Geometry: final body of the model. Coordinates: model frame, mm. Face numbers are marked on the shaded views. A direction names the side the tool comes from. Give positions to 0.01 mm unless a question says otherwise; leave off trailing zeros. Write each loop counter-clockwise with the first axis right and the second up, starting at its lowest first coordinate (ties: lowest second). Pieces come first, ordered by that corner, then holes. Notation, with made-up numbers: M 61.5,9 L 97.5,9 A34 cw 97.5,47 Z; hole C -18,0.25 d9. An arc over 180 degrees is marked long. Use a Markdown table: item, result. Add a question column.
1) Section A-A on x = 5. Return the cut outline in (y, z), then the cut area to 3 significant figures.
2) Section B-B on z = 5.5. Return the cut outline in (x, y).
3) Section C-C on x = -5.5. Return the cut outline in (y, z), then the cut area to 3 significant figures.
4) Line query: line 1 (Z direction, x = 5, y = 2.25); line 2 (Y direction, x = -5.5, z = 11); line 3 (Z direction, x = 3.5, y = 1.25). Output: solid intervals per line, ascending.
5) Draft query along X for the marked faces 3, 4, 5 and 6. Return one class per face: +X half, -X half, draft (parallel to the pull), parting line (faces both ways), or undercut.
6) Pin query (flat end, axial travel): pin 1 (4.5 mm diameter, centred on x = 5, z = 4.87, fed in from +Y); pin 2 (4 mm diameter, centred on x = -5.5, y = 4, fed in from -Z); pin 3 (1.5 mm diameter, centred on y = 4.5, z = 13, fed in from +X). Return the tip coordinate at first contact, or that it passes through.
7) Section D-D on z = 16.75. Return the cut outline in (x, y), then the cut area to 4 significant figures.
8) Set-up query: the marked faces 1 and 2. Return all of +Z, -Z, +X, -X, +Y, -Y with unobstructed straight access to the full face (end or side cutting, diameter ignored); none if empty.
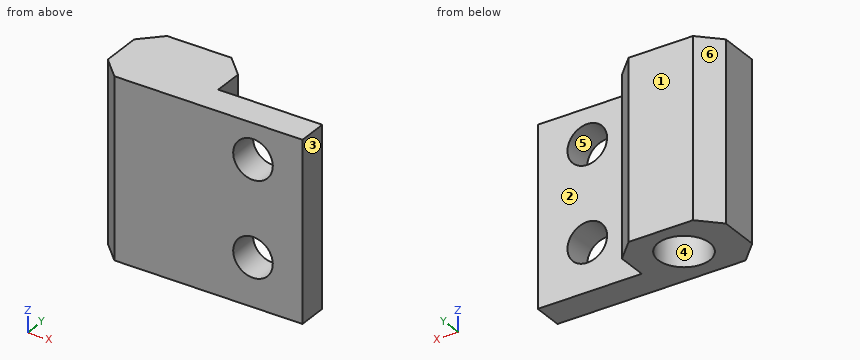
```python
from build123d import *

# Parameters (mm, degrees)
SKETCH_1_W          = 21
SKETCH_1_H          = 17.990855805
EXTRUDE_1_DEPTH     = 8
SKETCH_2_W          = 10.499999995
SKETCH_2_H          = 17.994369167
CUT_EXTRUDE_1_DEPTH = 5
SKETCH_3_R          = 1.999999882
SKETCH_3_R_2        = 1.999999942
CUT_EXTRUDE_2_DEPTH = 22.671891763
SKETCH_4_R          = 2.6
CUT_EXTRUDE_3_DEPTH = 15
CHAMFER_1_SIZE      = 2


with BuildPart() as part:
    # Эскиз1 → Вытянуть1 (new body)
    with BuildSketch(Plane(origin=(0, 0, 0), x_dir=(1, 0, 0), z_dir=(0, 1, 0))):
        with Locations((-0.5, -8.995427903)):
            Rectangle(SKETCH_1_W, SKETCH_1_H)
    extrude(amount=EXTRUDE_1_DEPTH)

    # Эскиз2 → Вырез-Вытянуть1 (cut)
    with BuildSketch(Plane(origin=(0, 8, 0), x_dir=(1, 0, 0), z_dir=(0, 1, 0))):
        with Locations((4.749999998, -8.993671222)):
            Rectangle(SKETCH_2_W, SKETCH_2_H)
    extrude(amount=-CUT_EXTRUDE_1_DEPTH, mode=Mode.SUBTRACT)

    # Эскиз3 → Вырез-Вытянуть2 (cut, through all)
    with BuildSketch(Plane(origin=(0, 3, 0), x_dir=(1, 0, 0), z_dir=(0, 1, 0))):
        with Locations(Location((4.999999995, -14.436118586, 0), (0, 0, 270))):
            Circle(SKETCH_3_R)
        with Locations(Location((4.999999995, -4.873583798, 0), (0, 0, 270))):
            Circle(SKETCH_3_R_2)
    extrude(amount=-CUT_EXTRUDE_2_DEPTH, mode=Mode.SUBTRACT)

    # Эскиз4 → Вырез-Вытянуть3 (cut)
    with BuildSketch(Plane.XY):
        with Locations((-5.500000032, 4.090743194)):
            Circle(SKETCH_4_R)
    extrude(amount=CUT_EXTRUDE_3_DEPTH, mode=Mode.SUBTRACT)

    # Фаска1
    chamfer_1_edges = [part.edges().sort_by_distance(p)[0] for p in [
        (-0.5, 8, 8.995427902),
        (-11, 8, 8.995427902),
        (-11, 0, 8.995427902),
    ]]
    chamfer(chamfer_1_edges, length=CHAMFER_1_SIZE)


solid = part.part
```
Found:
| question | item | result |
|---|---|---|
| 1 | outline | M 0,0 L 3,0 L 3,2.87 L 0,2.87 Z; M 0,6.87 L 3,6.87 L 3,12.44 L 0,12.44 Z; M 0,16.44 L 3,16.44 L 3,17.99 L 0,17.99 Z |
| 1 | area | 30.0 mm² |
| 2 | outline | M -11,2 L -9,0 L 3.1,0 L 3.1,3 L -0.5,3 L -0.5,6 L -2.5,8 L -9,8 L -11,6 Z; M 6.9,0 L 10,0 L 10,3 L 6.9,3 Z; hole C -5.5,4.09 d5.2 |
| 3 | outline | M 0,0 L 1.49,0 L 1.49,15 L 6.69,15 L 6.69,0 L 8,0 L 8,17.99 L 0,17.99 Z |
| 3 | area | 65.9 mm² |
| 4 | line 1 | 0 to 2.87, 6.87 to 12.44, 16.44 to 17.99 |
| 4 | line 2 | 0 to 1.49, 6.69 to 8 |
| 4 | line 3 | 0 to 3.55, 6.2 to 13.11, 15.76 to 17.99 |
| 5 | face 3 | +X half |
| 5 | face 4 | undercut |
| 5 | face 5 | undercut |
| 5 | face 6 | -X half |
| 6 | pin 1 | y = 3 |
| 6 | pin 2 | z = 15 |
| 6 | pin 3 | x = -0.5 |
| 7 | outline | M -11,2 L -9,0 L 10,0 L 10,3 L -0.5,3 L -0.5,6 L -2.5,8 L -9,8 L -11,6 Z |
| 7 | area | 109.5 mm² |
| 8 | face 1 | +Z, -Z, +X, -X, +Y |
| 8 | face 2 | +Z, -Z, +X, +Y |
